The listing builds one solid part. Answer for the finished solid, in the listing's coordinates (mm). A direction names the side the tool comes from. Give positions to 0.01 mm unless a question says otherwise; leave off trailing zeros. Write each loop counter-clockwise with the first axis right and the second up, starting at its lowest first coordinate (ties: lowest second). Pieces come first, ordered by that corner, then holes. Notation, with made-up numbers: (30.5, 66) - (38.5, 66) arc R19 ccw to (38.5, 92) - close; hole circle Ø1 at (68.25, 9). An arc over 180 degrees is marked (long way). One line per item, written item: value. Start each with the question number.
from build123d import *

# Parameters (mm, degrees)
F0_W     = 41.9582277536
F0_H     = 96.0698723793
F1_DEPTH = 45.72
F2_DEPTH = 47.244
F3_R     = 27.0129618135
F3_R_2   = 19.972912416
F4_DEPTH = 50.8
F5_DEPTH = 76.708


with BuildPart() as f1:
    # F0 (on Right) → F1 (new body)
    with BuildSketch(Plane.YZ):
        Rectangle(F0_W, F0_H)
    extrude(amount=F1_DEPTH)

    # F2 (add): a face of the model
    f2_faces = [f1.faces().sort_by_distance(p)[0] for p in [
        (0, 0, 0),
    ]]
    extrude(f2_faces, amount=F2_DEPTH)

    # F3 (on face) → F4 (join)
    with BuildSketch(Plane.XZ.offset(20.9791138768)):
        Circle(F3_R)
        Circle(F3_R_2, mode=Mode.SUBTRACT)
    extrude(amount=F4_DEPTH)

    # F5 (cut): a face of the model
    f5_faces = [f1.faces().sort_by_distance(p)[0] for p in [
        (0, -20.9791138768, 0),
    ]]
    extrude(f5_faces, amount=-F5_DEPTH, mode=Mode.SUBTRACT)


solid = f1.part
Item 1: For faces 1 (the cylindrical face through (25.766, -46.024, 8.114)), 2 (the flat face through (0, 0, -48.035)), determine the directions among +Z, -Z, +X, -X, +Y, -Y from which every point of the face is accessible in a straight line to the end or side of a thin tool.
Item 2: Find section B-B on x = 0. Determine the outline of the cut face in (y, z), plus the area to 3 significant figures.
Item 3: Find section D-D on x = -24. Determine the outline of the cut face in (y, z).
Item 4: Straight lines are drawn through the part: line 1 along Z through (x, y) = (0, -35); line 2 along Y through (x, z) = (-37.5, -11); line 3 along Z through (x, y) = (-4, 15). For each, find the intervals that lie inside material, in ascending order.
Item 5: Find section C-C on y = -9.5. Determine the outline of the cut face in (x, z), plus the area to 3 significant figures.
Item 6: Find section A-A on z = 0. Determine the outline of the cut face in (x, y), plus the area to 3 significant figures.
Item 7: Each of these flat-tipped pins is pushed along its axis until it touches: pin 1 Ø6 at (y, z) = (-54.5, -13) entering from -X; pin 2 Ø10 at (x, z) = (28, -4.5) entering from -Y; pin 3 Ø1.5 at (x, y) = (16.5, -29.5) entering from -Z; pin 4 Ø1.5 at (x, z) = (-19, -33) entering from -Y. Where does it stop, or does it pass through?
Values:
1. face 1: -Y
1. face 2: -Z, +X, -X, +Y, -Y
2. outline: (-71.78, -27.01) - (-20.98, -27.01) - (-20.98, -48.03) - (20.98, -48.03) - (20.98, -19.97) - (-71.78, -19.97) - close; (-71.78, 19.97) - (20.98, 19.97) - (20.98, 48.03) - (-20.98, 48.03) - (-20.98, 27.01) - (-71.78, 27.01) - close
2. area: 3,070 mm^2
3. outline: (-71.78, -12.4) - (-20.98, -12.4) - (-20.98, -48.03) - (20.98, -48.03) - (20.98, 48.03) - (-20.98, 48.03) - (-20.98, 12.4) - (-71.78, 12.4) - close
4. line 1: -27.01 to -19.97, 19.97 to 27.01
4. line 2: -20.98 to 20.98
4. line 3: -48.03 to -19.57, 19.57 to 48.03
5. outline: (-47.24, -48.03) - (45.72, -48.03) - (45.72, 48.03) - (-47.24, 48.03) - close; hole circle Ø39.95 at (0, 0)
5. area: 7,680 mm^2
6. outline: (-47.24, -20.98) - (-27.01, -20.98) - (-27.01, -71.78) - (-19.97, -71.78) - (-19.97, 20.98) - (-47.24, 20.98) - close; (19.97, -71.78) - (27.01, -71.78) - (27.01, -20.98) - (45.72, -20.98) - (45.72, 20.98) - (19.97, 20.98) - close
6. area: 2,940 mm^2
7. pin 1: x = -25.09
7. pin 2: y = -71.78
7. pin 3: z = -21.95
7. pin 4: y = -20.98
